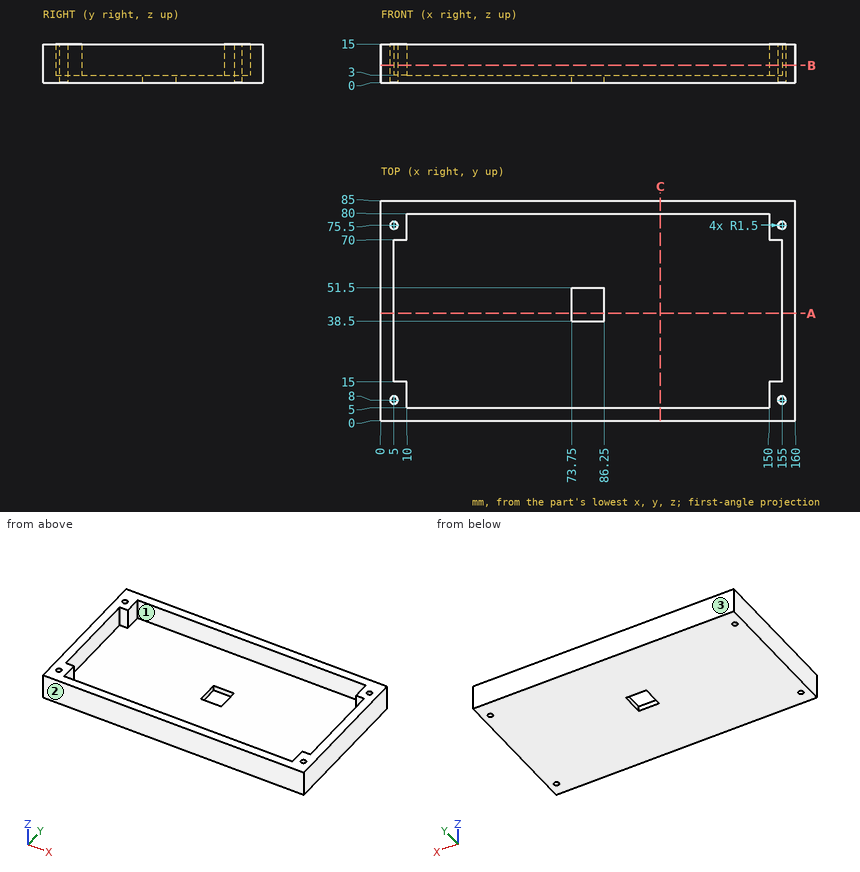
Design review of the part shown in the three views and the two pictorial views. Dimensions are in mm from the part's minimum x, y and z. Give positions to 0.01 mm unless a question says otherwise; leave off trailing zeros. Loops run counter-clockwise (first coordinate to the right, second up) from the corner with the lowest first, then second, coordinate; pieces in that order, holes last. Notation, with made-up numbers: M -0.75,78.5 L 6.25,78.5 A23 ccw 6.25,104.5 Z; hole C -17.75,0 d5. An arc over 180 degrees is marked long. Answer as a JSON object with one key per item and string values. Group by question number.
Q1. Add section B-B on z = 6.75. Give the boundary of the cut face in (x, y).
Q2. Insertion check: P1, Ø2, axis at x = 129, y = 51.5, coming from the +Z side. The pin has a flat end and moves straight along its axis. Give the tip position at first contact, or say it passes through.
Q3. Add section A-A on y = 41.5. Give the boundary of the cut face in (x, z), and give its area (4 significant figures).
Q4. For probe 1 along X at (y, z) = (16, 9.25); probe 2 along X at (y, z) = (48.5, 2.5); probe 3 along Y at (x, z) = (15, 4.5), list the stretches that pass through material, from the lowest coordinate up. Write a range as [from, to].
Q5. Add section C-C on x = 108. Give the boundary of the cut face in (y, z), and give its area (3 significant figures).
Q6. Mouldability with a two-part tool opening along Y and no side actions: class the marked faces 1, 2 and 3 as +Y half, -Y half, draft (parallel to the pull), parting line (faces both ways), or undercut.
Checked values:
{
 "1": {"outline": "M 0,0 L 160,0 L 160,85 L 0,85 Z; hole M 5,9.5 A1.5 ccw long 6.5,8 A1.5 ccw Z; hole M 5,15 L 10,15 L 10,5 L 150,5 L 150,15 L 155,15 L 155,70 L 150,70 L 150,80 L 10,80 L 10,70 L 5,70 Z; hole M 5,77 A1.5 ccw long 6.5,75.5 A1.5 ccw Z; hole M 155,9.5 A1.5 ccw long 156.5,8 A1.5 ccw Z; hole M 155,77 A1.5 ccw long 156.5,75.5 A1.5 ccw Z"},
 "2": {"P1": "z = 3"},
 "3": {"outline": "M 0,0 L 73.75,0 L 73.75,3 L 5,3 L 5,15 L 0,15 Z; M 86.25,0 L 160,0 L 160,15 L 155,15 L 155,3 L 86.25,3 Z", "area": "562.5 mm²"},
 "4": {"probe 1": "[0, 5], [155, 160]", "probe 2": "[0, 73.75], [86.25, 160]", "probe 3": "[0, 5], [80, 85]"},
 "5": {"outline": "M 0,0 L 85,0 L 85,15 L 80,15 L 80,3 L 5,3 L 5,15 L 0,15 Z", "area": "375 mm²"},
 "6": {"face 1": "undercut", "face 2": "-Y half", "face 3": "+Y half"}
}
